from build123d import *

# Parameters (mm, degrees)
AUFSATZ_LINEAR_AUSTRAGEN1_DEPTH      = 10
F_12_0_12_DURCHMESSER_BOHRUNG1_D     = 12
F_12_0_12_DURCHMESSER_BOHRUNG1_DEPTH = 30
F_12_0_12_DURCHMESSER_BOHRUNG1_TIP   = 3.605163714
M12_GEWINDEBOHRUNG1_D                = 10.2
M12_GEWINDEBOHRUNG1_DEPTH            = 32.75
M12_GEWINDEBOHRUNG1_TIP              = 3.064389157
SCHNITT_LINEAR_START                 = -10
SCHNITT_LINEAR_AUSTRAGEN1_OUTLINE_R  = 15.5
SCHNITT_LINEAR_AUSTRAGEN1_DEPTH      = 20
M10_START                            = -10
M10_GEWINDEBOHRUNG1_OUTLINE_R        = 4.25
M10_GEWINDEBOHRUNG1_DEPTH            = 20
M10_GEWINDEBOHRUNG2_D                = 8.5
M10_GEWINDEBOHRUNG2_DEPTH            = 27.5
M10_GEWINDEBOHRUNG2_TIP              = 2.553657631
FASE1_SIZE                           = 0.5


# Read off the part's stored shape, not the designer's step: Schnitt-Linear austragen1, M10 Gewindebohrung1
with BuildPart() as part:
    # Skizze1 → Aufsatz-Linear austragen1 (new, symmetric)
    with BuildSketch(Plane.XY):
        with BuildLine():
            Line((0, 0), (0, 420))
            Line((0, 420), (35, 420))
            ThreePointArc((35, 420), (42.653668647, 418.47759065), (49.142135624, 414.142135624))
            Line((49.142135624, 414.142135624), (379.142135624, 84.142135624))
            ThreePointArc((379.142135624, 84.142135624), (383.47759065, 77.653668647), (385, 70))
            Line((385, 70), (385, 20))
            ThreePointArc((385, 20), (379.142135624, 5.857864376), (365, 0))
            Line((365, 0), (0, 0))
        make_face()
    extrude(amount=AUFSATZ_LINEAR_AUSTRAGEN1_DEPTH, both=True)

    # Ø12.0 (12) Durchmesser Bohrung1
    with Locations(Plane.ZY):
        with Locations((0, 40), (0, 380)):
            Hole(F_12_0_12_DURCHMESSER_BOHRUNG1_D / 2, depth=F_12_0_12_DURCHMESSER_BOHRUNG1_DEPTH)
            with Locations((0, 0, -(F_12_0_12_DURCHMESSER_BOHRUNG1_DEPTH + F_12_0_12_DURCHMESSER_BOHRUNG1_TIP / 2))):  # 118° drill point
                Cone(0, F_12_0_12_DURCHMESSER_BOHRUNG1_D / 2, F_12_0_12_DURCHMESSER_BOHRUNG1_TIP, mode=Mode.SUBTRACT)

    # M12 Gewindebohrung1
    with Locations(Plane.ZY):
        with Locations((0, 20), (0, 210), (0, 400)):
            Hole(M12_GEWINDEBOHRUNG1_D / 2, depth=M12_GEWINDEBOHRUNG1_DEPTH)
            with Locations((0, 0, -(M12_GEWINDEBOHRUNG1_DEPTH + M12_GEWINDEBOHRUNG1_TIP / 2))):  # 118° drill point
                Cone(0, M12_GEWINDEBOHRUNG1_D / 2, M12_GEWINDEBOHRUNG1_TIP, mode=Mode.SUBTRACT)

    # Schnitt-Linear austragen1 outline → Schnitt-Linear austragen1 (cut)
    with BuildSketch(Plane.XY.offset(SCHNITT_LINEAR_START)):
        with BuildLine():
            Line((55, 277.389826945), (55, 72))
            ThreePointArc((55, 72), (61.443650814, 56.443650814), (77, 50))
            Line((77, 50), (258, 50))
            ThreePointArc((258, 50), (273.556349186, 56.443650814), (280, 72))
            Line((280, 72), (280, 96.389826945))
            ThreePointArc((280, 96.389826945), (278.325349715, 104.808862457), (273.556349186, 111.946176131))
            Line((273.556349186, 111.946176131), (92.556349186, 292.946176131))
            ThreePointArc((92.556349186, 292.946176131), (68.580964488, 297.71517666), (55, 277.389826945))
        make_face()
        with Locations((330, 70)):
            Circle(SCHNITT_LINEAR_AUSTRAGEN1_OUTLINE_R)
    extrude(amount=SCHNITT_LINEAR_AUSTRAGEN1_DEPTH, mode=Mode.SUBTRACT)

    # M10 Gewindebohrung1 outline → M10 Gewindebohrung1 (cut)
    with BuildSketch(Plane.XY.offset(M10_START)):
        with Locations((300.234254829, 120.07057933)):
            Circle(M10_GEWINDEBOHRUNG1_OUTLINE_R)
        with Locations((359.765745171, 19.92942067)):
            Circle(M10_GEWINDEBOHRUNG1_OUTLINE_R)
    extrude(amount=M10_GEWINDEBOHRUNG1_DEPTH, mode=Mode.SUBTRACT)

    # M10 Gewindebohrung2
    with Locations(Plane(origin=(0, 0, 0), x_dir=(-1, 0, 0), z_dir=(0, -1, 0))):
        with Locations((-324.5, 0), (-244.5, 0)):
            Hole(M10_GEWINDEBOHRUNG2_D / 2, depth=M10_GEWINDEBOHRUNG2_DEPTH)
            with Locations((0, 0, -(M10_GEWINDEBOHRUNG2_DEPTH + M10_GEWINDEBOHRUNG2_TIP / 2))):  # 118° drill point
                Cone(0, M10_GEWINDEBOHRUNG2_D / 2, M10_GEWINDEBOHRUNG2_TIP, mode=Mode.SUBTRACT)

    # Fase1
    fase1_edges = [part.edges().sort_by_distance(p)[0] for p in [
        (385, 45, 10),
        (379.142135624, 5.857864376, -10),
        (182.5, 0, -10),
        (383.47759065, 77.653668647, 10),
        (214.142135624, 249.142135624, 10),
        (42.653668647, 418.47759065, 10),
        (17.5, 420, 10),
        (182.5, 0, 10),
        (61.443650814, 56.443650814, -10),
        (55, 174.694913472, -10),
        (68.580964488, 297.71517666, -10),
        (183.056349186, 202.446176131, -10),
        (278.325349715, 104.808862457, -10),
        (280, 84.194913472, -10),
        (273.556349186, 56.443650814, -10),
        (167.5, 50, -10),
        (61.443650814, 56.443650814, 10),
        (167.5, 50, 10),
        (273.556349186, 56.443650814, 10),
        (280, 84.194913472, 10),
        (278.325349715, 104.808862457, 10),
        (183.056349186, 202.446176131, 10),
        (68.580964488, 297.71517666, 10),
        (55, 174.694913472, 10),
        (379.142135624, 5.857864376, 10),
        (314.5, 70, -10),
        (314.5, 70, 10),
        (17.5, 420, -10),
        (42.653668647, 418.47759065, -10),
        (214.142135624, 249.142135624, -10),
        (383.47759065, 77.653668647, -10),
        (385, 45, -10),
    ]]
    chamfer(fase1_edges, length=FASE1_SIZE)


solid = part.part
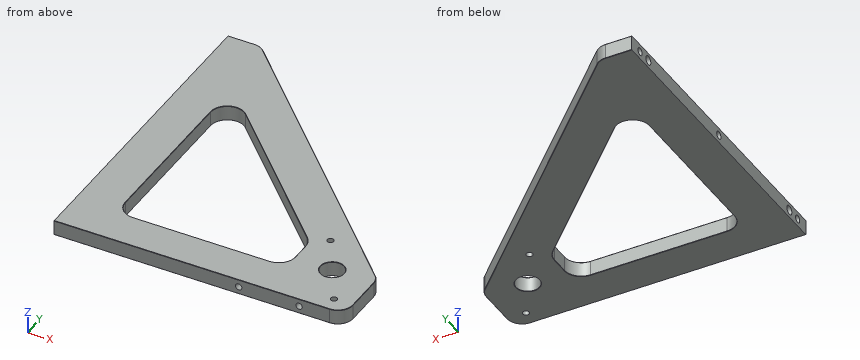
Input: part model. Units: mm. Frame: model coordinates. Give positions to 0.01 mm unless a question says otherwise; leave off trailing zeros. Order: outer loops, then holes, each group sorted by start corner. A loop starts at its lowest first (then second) coordinate and runs counter-clockwise, first axis right, second up.
Q1. Ray query, probe 1 along Y at (x, z) = (10, 0); probe 2 along Z at (x, y) = (11.25, 40); probe 3 along Z at (x, y) = (244, 17). Return the intervals inside material, ascending.
Checked values:
probe 1: y = 0 to 14.9, 25.1 to 34, 46 to 204.9, 215.1 to 374, 386 to 394.9, 405.1 to 420
probe 2: z = -10 to -6, 6 to 10
probe 3: z = -10 to -4.22, 4.22 to 10
Q2. Section A-A on y = 136. Output: boundary loops of the cut face in (x, z), and give its area (3 significant figures).
Checked values:
outline: (0, -10) - (54.5, -10) - (55, -9.5) - (55, 9.5) - (54.5, 10) - (0, 10) - close; (249.5, -9.5) - (250.21, -10) - (326.58, -10) - (327.28, -9.5) - (327.28, 9.5) - (326.58, 10) - (250.21, 10) - (249.5, 9.5) - close
area: 2,650 mm2
Q3. Contact query for flat-ended pins moving along their axis: pin 1 Ø18.5 at (x, y) = (330, 70) entering from +Z; pin 2 Ø7 at (x, z) = (244.5, 0) entering from +Y; pin 3 Ø11.5 at (y, z) = (400, 0) entering from +X; pin 4 Ø11 at (y, z) = (380, 0) entering from -X. Output: stop coordinate, or through.
Checked values:
pin 1: passes through
pin 2: stops at y = 222.28
pin 3: stops at x = 69.03
pin 4: stops at x = 30.3
